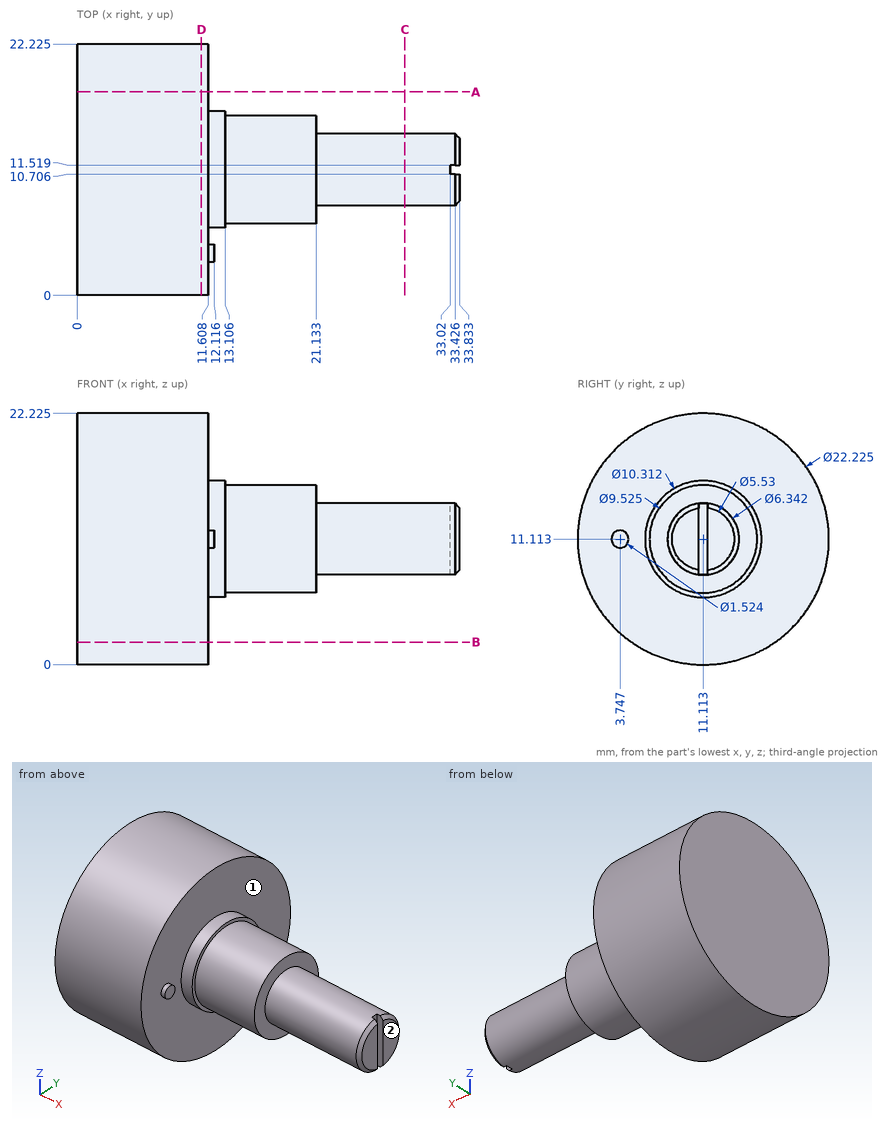
Study the drawing (mm; zero at the part's minimum x, y, z) and answer. A direction names the side the tool comes from. Round coordinates to 2 decimals unless told otherwise and drop trailing zeros. Write each loop counter-clockwise with the first axis right and the second up, starting at its lowest first coordinate (ties: lowest second). Pieces come first, ordered by that corner, then holes.
Q1. Straight lines are drawn through the part: line 1 (X direction, y = 7, z = 6); line 2 (Y direction, x = 23, z = 11); line 3 (Y direction, x = 22.5, z = 10.75). For each, find the intervals that lie inside material, in ascending order.
Values:
line 1: x = 0 to 11.61
line 2: y = 7.94 to 14.28
line 3: y = 7.96 to 14.26
Q2. Find section C-C on x = 29. Determine the outline of the cut face in (y, z), and give its area (3 significant figures).
Values:
outline: circle Ø6.34 at (11.11, 11.11)
area: 31.6 mm2
Q3. A tool of negligible diameter and unlimited length cuts with its end or side. For the marked faces 1 and 2, from which of +Z, -Z, +X, -X, +Y, -Y can it reach the whole face along a straight path? Write none if from no direction.
Values:
face 1: +X
face 2: +Z, -Z, +X, +Y, -Y
Q4. Find section D-D on x = 11. Determine the outline of the cut face in (y, z) (1 decimal), and give its area (3 significant figures).
Values:
outline: circle Ø22.2 at (11.1, 11.1)
area: 388 mm2
Q5. Find section A-A on y = 18. Determine the outline of the cut face in (x, z).
Values:
outline: (0, 2.39) - (11.61, 2.39) - (11.61, 19.83) - (0, 19.83) - close
Q6. Find section B-B on z = 2. Determine the outline of the cut face in (x, y), and give its area (3 significant figures).
Values:
outline: (0, 4.75) - (11.61, 4.75) - (11.61, 17.47) - (0, 17.47) - close
area: 148 mm2
Q7. Flat-ended cylindrical pins translate along their axes: P1, Ø10, axis at y = 18.5, z = 4, coming from the +X side; P2, Ø4, axis at x = 30, y = 13, coming from the -Z side; P3, Ø1.5, axis at x = 12, y = 10, coming from the -Z side. Find the tip coordinate at first contact, or state that the pin passes through.
Values:
P1: stops at x = 11.61
P2: stops at z = 7.94
P3: stops at z = 0.01
